For this review, take the finished solid that the model builds, in its own axes (mm). A direction names the side the tool comes from. Round coordinates to 2 decimals unless told otherwise and drop trailing zeros. Write each loop counter-clockwise with the first axis right and the second up, starting at its lowest first coordinate (ties: lowest second). Pieces come first, ordered by that corner, then holes. Notation, with made-up numbers: (67.5, -39.75) - (91.5, -39.75) arc R21 ccw to (91.5, -35.75) - close; hole circle Ø1 at (4, 3.5). An arc over 180 degrees is marked (long way). Answer in a Markdown table with one row per item. Add a question column.
from build123d import *

# Parameters (mm, degrees)
SKETCH1_W                       = 40
SKETCH1_H                       = 35
BOSS_EXTRUDE1_DEPTH             = 18
CAVITY1_START                   = -14.401086919
CAVITY1_OUTLINE_W               = 23
CAVITY1_OUTLINE_H               = 12
CAVITY1_DEPTH                   = 21.5
CAVITY1_START_2                 = 7.098913081
CAVITY1_2_OUTLINE_R             = 5
CAVITY1_2_DEPTH                 = 3
CAVITY1_START_3                 = 1.098913081
CAVITY1_3_DEPTH                 = 2
CAVITY1_START_4                 = 10.098913081
CAVITY1_4_OUTLINE_R             = 2.5
CAVITY1_4_DEPTH                 = 4
CUT_EXTRUDE1_DEPTH              = 42.733432002
CUT_EXTRUDE1_DEPTH_BACK         = 42.733432002
SKETCH2_W                       = 52.530025258
SKETCH2_H                       = 12.54309889
CUT_EXTRUDE2_DEPTH              = 43
SKETCH4_W                       = 40
SKETCH4_H                       = 7.548254148
CUT_EXTRUDE3_DEPTH              = 43
BOSS_EXTRUDE2_DEPTH             = 3
SKETCH6_W                       = 81.743347259
SKETCH6_H                       = 13.911125845
BOSS_EXTRUDE3_DEPTH             = 10
SKETCH8_W                       = 4.746846532
SKETCH8_H                       = 29.399300547
BOSS_EXTRUDE4_DEPTH             = 20
BOSS_EXTRUDE4_DIRECTION_2_REACH = 67.288
SKETCH9_R                       = 2
CUT_EXTRUDE4_DEPTH              = 34
SKETCH10_R                      = 4
SKETCH10_R_2                    = 2
BOSS_EXTRUDE5_DEPTH             = 7
BOSS_EXTRUDE6_DEPTH             = 5.186094658
BOSS_EXTRUDE7_DEPTH             = 12
SKETCH14_W                      = 81.743347259
SKETCH14_H                      = 8.25177529
BOSS_EXTRUDE8_DEPTH             = 20
SKETCH16_W                      = 140.221979832
SKETCH16_H                      = 55
BOSS_EXTRUDE9_DEPTH             = 8.25
SKETCH17_R                      = 5
CUT_EXTRUDE5_DEPTH              = 10


# Read off the part's stored shape, not the designer's step: Cavity1
with BuildPart() as part:
    # Sketch1 → Boss-Extrude1 (new body)
    with BuildSketch(Plane(origin=(0, 0, 0), x_dir=(1, 0, 0), z_dir=(0, 1, 0))):
        Rectangle(SKETCH1_W, SKETCH1_H)
    extrude(amount=BOSS_EXTRUDE1_DEPTH)

    # Cavity1 outline → Cavity1 (cut)
    with BuildSketch(Plane.XY.offset(CAVITY1_START)):
        with Locations((0, 9)):
            Rectangle(CAVITY1_OUTLINE_W, CAVITY1_OUTLINE_H)
    extrude(amount=CAVITY1_DEPTH, mode=Mode.SUBTRACT)

    # Cavity1 2 outline → Cavity1 2 (cut)
    with BuildSketch(Plane.XY.offset(CAVITY1_START_2)):
        with Locations((5.5, 9)):
            Circle(CAVITY1_2_OUTLINE_R)
    extrude(amount=CAVITY1_2_DEPTH, mode=Mode.SUBTRACT)

    # Cavity1 3 outline → Cavity1 3 (cut)
    with BuildSketch(Plane.XY.offset(CAVITY1_START_3)):
        with BuildLine():
            Line((-11.5, 15), (-16, 15))
            Line((-16, 15), (-16, 10.821261352))
            Line((-16, 10.821261352), (-14.337589365, 10.821261352))
            ThreePointArc((-14.337589365, 10.821261352), (-12.516328014, 9), (-14.337589365, 7.178738648))
            Line((-14.337589365, 7.178738648), (-16, 7.178738648))
            Line((-16, 7.178738648), (-16, 3))
            Line((-16, 3), (-11.5, 3))
            Line((-11.5, 3), (-11.5, 15))
        make_face()
        with BuildLine():
            Line((16, 15), (11.5, 15))
            Line((11.5, 15), (11.5, 3))
            Line((11.5, 3), (16, 3))
            Line((16, 3), (16, 7.178738648))
            Line((16, 7.178738648), (14.337589365, 7.178738648))
            ThreePointArc((14.337589365, 7.178738648), (12.516328014, 9), (14.337589365, 10.821261352))
            Line((14.337589365, 10.821261352), (16, 10.821261352))
            Line((16, 10.821261352), (16, 15))
        make_face()
    extrude(amount=CAVITY1_3_DEPTH, mode=Mode.SUBTRACT)

    # Cavity1 4 outline → Cavity1 4 (cut)
    with BuildSketch(Plane.XY.offset(CAVITY1_START_4)):
        with Locations((5.5, 9)):
            Circle(CAVITY1_4_OUTLINE_R)
    extrude(amount=CAVITY1_4_DEPTH, mode=Mode.SUBTRACT)

    # Sketch2 → Cut-Extrude1 (cut, two sides: drawn at the far end of the back side and taken through both)
    with BuildSketch(Plane.XY.offset(-14.401086919).offset(-CUT_EXTRUDE1_DEPTH_BACK)):
        with Locations((5.5, 15.271549445)):
            Rectangle(SKETCH2_W, SKETCH2_H)
    extrude(amount=CUT_EXTRUDE1_DEPTH + CUT_EXTRUDE1_DEPTH_BACK, mode=Mode.SUBTRACT)

    # Sketch3 → Cut-Extrude2 (cut)
    with BuildSketch(Plane(origin=(0, 3, 0), x_dir=(1, 0, 0), z_dir=(0, 1, 0))):
        Polygon((-11.5, -3.098913081), (-11.5, -7.098913081), (11.5, -7.098913081), (11.5, -3.098913081), (16, -3.098913081), (16, -1.098913081), (11.5, -1.098913081), (11.5, 14.401086919), (-11.5, 14.401086919), (-11.5, -1.098913081), (-16, -1.098913081), (-16, -3.098913081), align=None)
    extrude(amount=CUT_EXTRUDE2_DEPTH, mode=Mode.SUBTRACT)

    # Sketch4 → Cut-Extrude3 (cut)
    with BuildSketch(Plane(origin=(0, 9, 0), x_dir=(1, 0, 0), z_dir=(0, 1, 0))):
        with Locations((0, -13.725872926)):
            Rectangle(SKETCH4_W, SKETCH4_H)
    extrude(amount=-CUT_EXTRUDE3_DEPTH, mode=Mode.SUBTRACT)

    # Sketch5 → Boss-Extrude2 (add)
    with BuildSketch(Plane(origin=(0, 9, 0), x_dir=(1, 0, 0), z_dir=(0, 1, 0))):
        Polygon((10.5, -9.951745852), (20, -9.951745852), (20, 17.5), (-20, 17.5), (-20, -9.951745852), (0.5, -9.951745852), (0.5, -7.098913081), (-11.5, -7.098913081), (-11.5, -3.098913081), (-16, -3.098913081), (-16, -1.098913081), (-11.5, -1.098913081), (-11.5, 14.401086919), (11.5, 14.401086919), (11.5, -1.098913081), (16, -1.098913081), (16, -3.098913081), (11.5, -3.098913081), (11.5, -7.098913081), (10.5, -7.098913081), align=None)
    extrude(amount=BOSS_EXTRUDE2_DEPTH)

    # Sketch6 → Boss-Extrude3 (add)
    with BuildSketch(Plane.XZ):
        with Locations((-20.87167363, -5.358342419)):
            Rectangle(SKETCH6_W, SKETCH6_H)
    extrude(amount=BOSS_EXTRUDE3_DEPTH)

    # Sketch8 → Boss-Extrude4 (add)
    with BuildSketch(Plane(origin=(0, 0, 0), x_dir=(1, 0, 0), z_dir=(0, 1, 0))):
        with Locations((-59.369923993, -2.385744932)):
            Rectangle(SKETCH8_W, SKETCH8_H)
        with Locations((-50.602645133, -2.385744932)):
            Rectangle(SKETCH8_W, SKETCH8_H)
    extrude(amount=BOSS_EXTRUDE4_DEPTH)

    # Boss-Extrude4 direction 2: up to this face of the body (flat: up to its plane)
    boss_extrude4_direction_2_end = Plane(part.part.faces().sort_by_distance((-20.87167363, -10, -5.358342419))[0])
    # Sketch8 → Boss-Extrude4 direction 2 (add, up to the picked face)
    with BuildSketch(Plane(origin=(0, 0, 0), x_dir=(1, 0, 0), z_dir=(0, 1, 0)), mode=Mode.PRIVATE) as boss_extrude4_direction_2_sk1:
        with Locations((-59.369923993, -2.385744932)):
            Rectangle(SKETCH8_W, SKETCH8_H)
    boss_extrude4_direction_2_tool1 = split(extrude(boss_extrude4_direction_2_sk1.sketch, amount=-BOSS_EXTRUDE4_DIRECTION_2_REACH, mode=Mode.PRIVATE), bisect_by=boss_extrude4_direction_2_end, keep=Keep.BOTH, mode=Mode.PRIVATE)
    # Sketch8 → Boss-Extrude4 direction 2 (add, up to the picked face)
    with BuildSketch(Plane(origin=(0, 0, 0), x_dir=(1, 0, 0), z_dir=(0, 1, 0)), mode=Mode.PRIVATE) as boss_extrude4_direction_2_sk2:
        with Locations((-50.602645133, -2.385744932)):
            Rectangle(SKETCH8_W, SKETCH8_H)
    boss_extrude4_direction_2_tool2 = split(extrude(boss_extrude4_direction_2_sk2.sketch, amount=-BOSS_EXTRUDE4_DIRECTION_2_REACH, mode=Mode.PRIVATE), bisect_by=boss_extrude4_direction_2_end, keep=Keep.BOTH, mode=Mode.PRIVATE)
    add(boss_extrude4_direction_2_tool1.solids().sort_by(Axis((-59.369924, 0, 2.385745), (0, -1, 0)))[0])
    add(boss_extrude4_direction_2_tool2.solids().sort_by(Axis((-50.602645, 0, 2.385745), (0, -1, 0)))[0])

    # Sketch9 → Cut-Extrude4 (cut)
    with BuildSketch(Plane.ZY.offset(61.743347259)):
        with Locations((13.051745852, 14.536175319)):
            Circle(SKETCH9_R)
    extrude(amount=-CUT_EXTRUDE4_DEPTH, mode=Mode.SUBTRACT)

    # Sketch10 → Boss-Extrude5 (add)
    with BuildSketch(Plane(origin=(-48.229221867, 0, 0), x_dir=(0, 0, -1), z_dir=(1, 0, 0))):
        with Locations((-13.051745852, 14.536175319)):
            Circle(SKETCH10_R)
        with Locations(Location((-13.051745852, 14.536175319, 0), (0, 0, 180))):
            Circle(SKETCH10_R_2, mode=Mode.SUBTRACT)
    extrude(amount=BOSS_EXTRUDE5_DEPTH)

    # Sketch11 → Boss-Extrude6 (add)
    with BuildSketch(Plane(origin=(0, 0, -12.313905342), x_dir=(-1, 0, 0), z_dir=(0, 0, -1))):
        Polygon((61.743347259, -10), (61.743347259, 20), (56.996500727, 20), (56.996500727, 0), (52.976068399, 0), (52.976068399, 20), (48.229221867, 20), (48.229221867, 0), (20, 0), (-20, 0), (-20, -10), align=None)
    extrude(amount=BOSS_EXTRUDE6_DEPTH)

    # Sketch12 → Boss-Extrude7 (add)
    with BuildSketch(Plane(origin=(0, 0, -17.5), x_dir=(-1, 0, 0), z_dir=(0, 0, -1))):
        Polygon((20, 0), (20, 12), (-20, 12), (-20, -10), (61.743347259, -10), (61.743347259, 20), (56.996500727, 20), (56.996500727, 0), (52.976068399, 0), (52.976068399, 20), (48.229221867, 20), (48.229221867, 0), align=None)
    extrude(amount=BOSS_EXTRUDE7_DEPTH)

    # Sketch14 → Boss-Extrude8 (add)
    with BuildSketch(Plane(origin=(0, 0, 0), x_dir=(1, 0, 0), z_dir=(0, 1, 0))):
        with Locations((-20.87167363, 25.374112355)):
            Rectangle(SKETCH14_W, SKETCH14_H)
    extrude(amount=BOSS_EXTRUDE8_DEPTH)

    # Sketch16 → Boss-Extrude9 (add)
    with BuildSketch(Plane(origin=(0, 0, -29.5), x_dir=(-1, 0, 0), z_dir=(0, 0, -1))):
        with Locations((20.535780022, 5)):
            Rectangle(SKETCH16_W, SKETCH16_H)
    extrude(amount=-BOSS_EXTRUDE9_DEPTH)

    # Sketch17 → Cut-Extrude5 (cut)
    with BuildSketch(Plane(origin=(0, 0, -29.5), x_dir=(-1, 0, 0), z_dir=(0, 0, -1))):
        with Locations((-29.464219978, 25)):
            Circle(SKETCH17_R)
        with Locations((-29.464219978, -15)):
            Circle(SKETCH17_R)
        with Locations((70.535780022, 25)):
            Circle(SKETCH17_R)
        with Locations((70.535780022, -15)):
            Circle(SKETCH17_R)
    extrude(amount=-CUT_EXTRUDE5_DEPTH, mode=Mode.SUBTRACT)


solid = part.part
Q1. Add section C-C on y = -7.5. State the section outline as (x, z) points, then the cut area to 3 significant figures.
Q2. To check wall thickness, follow probe 1 along X at (y, z) = (11.5, -9); probe 2 along X at (y, z) = (1, -16.5); probe 3 along X at (y, z) = (19, 14). State the ranges of each line that lie inside material, in increasing order.
Q3. Tool access review of faces 5 (the face through (10.5, 10, 9)), 6 (the face through (-14, 7, 3.099)), 7 (the face through (0, 0, 6)): name each direction out of +Z, -Z, +X, -X, +Y, -Y from which nothing blocks a thin tool from reaching the whole face with its end or side.
Q4. Add section B-B on y = -15. State the section outline as (x, z) points.
Q5. Draft analysis for pull direction Z (two halves, no side actions). For faces 1 (the face through (-51, 5, 17.085)), 2 (the face through (11.5, 7, -7)), 3 (the face through (-20, 5, -29.5)), 4 (the face through (14, 7, 3.099)), state which applies: released by +Z, released by -Z, zero draft, split by the parting line, or undercut.
Q6. Insertion check: pin 1 Ø18.5 at (x, z) = (-28, -13) entering from +Y; pin 2 Ø6 at (y, z) = (-4.5, -6.5) entering from +X; pin 3 Ø10 at (x, y) = (-5.5, 9) entering from +Z; pin 4 Ø3 at (x, y) = (-55, 11.5) entering from +Z. Each pin has a flat end and moves straight along its axis. Give the tip position at first contact, or say it passes through.
Q7. Add section A-A on z = 5.5. State the section outline as (x, y) points.
Answer sheet:
| question | item | result |
|---|---|---|
| 1 | outline | (-90.65, -29.5) - (49.58, -29.5) - (49.58, -21.25) - (20, -21.25) - (20, 1.6) - (-48.23, 1.6) - (-48.23, 17.09) - (-52.98, 17.09) - (-52.98, 1.6) - (-57, 1.6) - (-57, 17.09) - (-61.74, 17.09) - (-61.74, -21.25) - (-90.65, -21.25) - close |
| 1 | area | 3,170 mm² |
| 2 | probe 1 | x = -61.74 to -57, -52.98 to -48.23, -20 to -11.5, 11.5 to 20 |
| 2 | probe 2 | x = -61.74 to -57, -52.98 to -48.23, -20 to 20 |
| 2 | probe 3 | x = -61.74 to -57, -52.98 to -48.23 |
| 3 | face 5 | +Z, +Y |
| 3 | face 6 | +Y |
| 3 | face 7 | +Z, +X, -Y |
| 4 | outline | (-90.65, -29.5) - (-75.54, -29.5) - (-75.54, -21.25) - (-90.65, -21.25) - close; (-65.54, -29.5) - (24.46, -29.5) - (24.46, -21.25) - (-65.54, -21.25) - close; (34.46, -29.5) - (49.58, -29.5) - (49.58, -21.25) - (34.46, -21.25) - close |
| 5 | face 1 | released by +Z |
| 5 | face 2 | undercut |
| 5 | face 3 | released by -Z |
| 5 | face 4 | undercut |
| 6 | pin 1 | stops at y = 32.5 |
| 6 | pin 2 | stops at x = 20 |
| 6 | pin 3 | stops at z = 9.95 |
| 6 | pin 4 | stops at z = -21.25 |
| 7 | outline | (-61.74, -10) - (-57, -10) - (-57, 20) - (-61.74, 20) - close; (-52.98, -10) - (-48.23, -10) - (-48.23, 20) - (-52.98, 20) - close; (-20, 0) - (20, 0) - (20, 12) - (11.5, 12) - (11.5, 3) - (-11.5, 3) - (-11.5, 12) - (-20, 12) - close |
